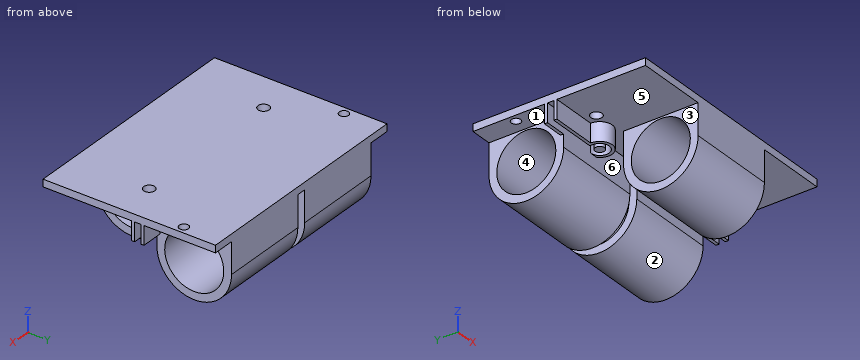
from build123d import *

# Parameters (mm, degrees)
SKETCH1_R              = 1.79994
SKETCH1_R_2            = 1.5
BOSS_EXTRUDE1_DEPTH    = 7
SKETCH2_W              = 75
SKETCH2_H              = 13.099999962
SKETCH2_R              = 2.6999438
SKETCH2_R_2            = 2.499995
SKETCH2_R_3            = 1.3498449
BOSS_EXTRUDE2_DEPTH    = 6.987999994
SKETCH2_3_R            = 2.6999438
SKETCH2_3_R_2          = 1.3498449
CUT_EXTRUDE1_DEPTH     = 2.5
SKETCH5_W              = 75
SKETCH5_H              = 13.099999962
CUT_EXTRUDE3_DEPTH     = 21.082
SKETCH6_W              = 75
SKETCH6_H              = 7
BOSS_EXTRUDE3_DEPTH    = 9.5
SKETCH8_W              = 75
SKETCH8_H              = 38.030205227
CUT_EXTRUDE4_DEPTH     = 4.666
SKETCH10_W             = 75
SKETCH10_H             = 2.334
BOSS_EXTRUDE5_DEPTH    = 25.000000038
SKETCH11_R             = 1.79994
CUT_EXTRUDE5_DEPTH     = 5
SKETCH15_W             = 44.653530321
SKETCH15_H             = 13.617301916
SKETCH15_W_2           = 11.728266088
SKETCH15_H_2           = 5.987537529
BOSS_EXTRUDE7_DEPTH    = 2.334
SKETCH16_R             = 9.5
BOSS_EXTRUDE9_DEPTH    = 29
SKETCH17_R             = 9.5
BOSS_EXTRUDE11_DEPTH   = 14.5
SKETCH18_W             = 6.99999997
SKETCH18_H             = 1
BOSS_EXTRUDE12_DEPTH   = 6
BOSS_EXTRUDE12_2_DEPTH = 6
SKETCH18_R             = 1.5
BOSS_EXTRUDE12_3_DEPTH = 6


with BuildPart() as part:
    # Sketch1 → Boss-Extrude1 (new body)
    with BuildSketch(Plane.XY):
        with BuildLine():
            Line((37.5, -10.5), (30, -10.5))
            ThreePointArc((30, -10.5), (25, -15.5), (20, -10.5))
            Line((20, -10.5), (5, -10.5))
            ThreePointArc((5, -10.5), (0, -15.5), (-5, -10.5))
            Line((-5, -10.5), (-20, -10.5))
            ThreePointArc((-20, -10.5), (-25, -15.5), (-30, -10.5))
            Line((-30, -10.5), (-37.5, -10.5))
            Line((-37.5, -10.5), (-37.5, 10.5))
            Line((-37.5, 10.5), (37.5, 10.5))
            Line((37.5, 10.5), (37.5, -10.5))
        make_face()
        with Locations((-25, -10.5)):
            Circle(SKETCH1_R, mode=Mode.SUBTRACT)
        with Locations((0, -10.5)):
            Circle(SKETCH1_R, mode=Mode.SUBTRACT)
        with Locations((25, -10.5)):
            Circle(SKETCH1_R, mode=Mode.SUBTRACT)
        with Locations((-35, 8)):
            Circle(SKETCH1_R_2, mode=Mode.SUBTRACT)
        with Locations(Location((-15, 8, 0), (0, 0, 180))):
            Circle(SKETCH1_R_2, mode=Mode.SUBTRACT)
        with Locations((-10, 8)):
            Circle(SKETCH1_R_2, mode=Mode.SUBTRACT)
        with Locations(Location((10, 8, 0), (0, 0, 180))):
            Circle(SKETCH1_R_2, mode=Mode.SUBTRACT)
        with Locations(Location((35, 8, 0), (0, 0, 180))):
            Circle(SKETCH1_R_2, mode=Mode.SUBTRACT)
        with Locations((15, 8)):
            Circle(SKETCH1_R_2, mode=Mode.SUBTRACT)
    extrude(amount=BOSS_EXTRUDE1_DEPTH)

    # Sketch2 → Boss-Extrude2 (add)
    # profile 1 of 7: a face of its own
    with BuildSketch(Plane(origin=(0, 2.24999999, 0), x_dir=(1, 0, 0), z_dir=(0, 1, 0))):
        with Locations((0, -13.549999981)):
            Rectangle(SKETCH2_W, SKETCH2_H)
        with Locations((31.0001404, -13.549999981)):
            Circle(SKETCH2_R, mode=Mode.SUBTRACT)
        with Locations((-31.0001404, -13.549999981)):
            Circle(SKETCH2_R, mode=Mode.SUBTRACT)
        with Locations(Location((-25, -13.549999981, 0), (0, 0, 180))):
            Circle(SKETCH2_R_2, mode=Mode.SUBTRACT)
        with Locations((-6.0001404, -13.549999981)):
            Circle(SKETCH2_R, mode=Mode.SUBTRACT)
        with Locations((6.0001404, -13.549999981)):
            Circle(SKETCH2_R, mode=Mode.SUBTRACT)
        with Locations(Location((0, -13.549999981, 0), (0, 0, 180))):
            Circle(SKETCH2_R_2, mode=Mode.SUBTRACT)
        with Locations((-18.9998596, -13.549999981)):
            Circle(SKETCH2_R, mode=Mode.SUBTRACT)
        with Locations(Location((25, -13.549999981, 0), (0, 0, 180))):
            Circle(SKETCH2_R_2, mode=Mode.SUBTRACT)
        with Locations((18.9998596, -13.549999981)):
            Circle(SKETCH2_R, mode=Mode.SUBTRACT)
    # profile 2 of 7: a face of its own
    with BuildSketch(Plane(origin=(0, 2.24999999, 0), x_dir=(1, 0, 0), z_dir=(0, 1, 0))):
        with Locations((-31.0001404, -13.549999981)):
            Circle(SKETCH2_R)
        with Locations(Location((-31.0001404, -13.549999981, 0), (0, 0, 180))):
            Circle(SKETCH2_R_3, mode=Mode.SUBTRACT)
    # profile 3 of 7: a face of its own
    with BuildSketch(Plane(origin=(0, 2.24999999, 0), x_dir=(1, 0, 0), z_dir=(0, 1, 0))):
        with Locations((-18.9998596, -13.549999981)):
            Circle(SKETCH2_R)
        with Locations(Location((-18.9998596, -13.549999981, 0), (0, 0, 180))):
            Circle(SKETCH2_R_3, mode=Mode.SUBTRACT)
    # profile 4 of 7: a face of its own
    with BuildSketch(Plane(origin=(0, 2.24999999, 0), x_dir=(1, 0, 0), z_dir=(0, 1, 0))):
        with Locations((-6.0001404, -13.549999981)):
            Circle(SKETCH2_R)
        with Locations(Location((-6.0001404, -13.549999981, 0), (0, 0, 180))):
            Circle(SKETCH2_R_3, mode=Mode.SUBTRACT)
    # profile 5 of 7: a face of its own
    with BuildSketch(Plane(origin=(0, 2.24999999, 0), x_dir=(1, 0, 0), z_dir=(0, 1, 0))):
        with Locations((6.0001404, -13.549999981)):
            Circle(SKETCH2_R)
        with Locations(Location((6.0001404, -13.549999981, 0), (0, 0, 180))):
            Circle(SKETCH2_R_3, mode=Mode.SUBTRACT)
    # profile 6 of 7: a face of its own
    with BuildSketch(Plane(origin=(0, 2.24999999, 0), x_dir=(1, 0, 0), z_dir=(0, 1, 0))):
        with Locations((18.9998596, -13.549999981)):
            Circle(SKETCH2_R)
        with Locations(Location((18.9998596, -13.549999981, 0), (0, 0, 180))):
            Circle(SKETCH2_R_3, mode=Mode.SUBTRACT)
    # profile 7 of 7: a face of its own
    with BuildSketch(Plane(origin=(0, 2.24999999, 0), x_dir=(1, 0, 0), z_dir=(0, 1, 0))):
        with Locations((31.0001404, -13.549999981)):
            Circle(SKETCH2_R)
        with Locations(Location((31.0001404, -13.549999981, 0), (0, 0, 180))):
            Circle(SKETCH2_R_3, mode=Mode.SUBTRACT)
    extrude(amount=-BOSS_EXTRUDE2_DEPTH)

    # Sketch2<3> → Cut-Extrude1 (cut)
    # profile 1 of 6: a face of its own
    with BuildSketch(Plane(origin=(0, 2.24999999, 0), x_dir=(1, 0, 0), z_dir=(0, 1, 0))):
        with Locations(Location((-31.0001404, -13.549999981, 0), (0, 0, 180))):
            Circle(SKETCH2_3_R)
        with Locations(Location((-31.0001404, -13.549999981, 0), (0, 0, 180))):
            Circle(SKETCH2_3_R_2, mode=Mode.SUBTRACT)
    # profile 2 of 6: a face of its own
    with BuildSketch(Plane(origin=(0, 2.24999999, 0), x_dir=(1, 0, 0), z_dir=(0, 1, 0))):
        with Locations(Location((-18.9998596, -13.549999981, 0), (0, 0, 180))):
            Circle(SKETCH2_3_R)
        with Locations(Location((-18.9998596, -13.549999981, 0), (0, 0, 180))):
            Circle(SKETCH2_3_R_2, mode=Mode.SUBTRACT)
    # profile 3 of 6: a face of its own
    with BuildSketch(Plane(origin=(0, 2.24999999, 0), x_dir=(1, 0, 0), z_dir=(0, 1, 0))):
        with Locations(Location((-6.0001404, -13.549999981, 0), (0, 0, 180))):
            Circle(SKETCH2_3_R)
        with Locations(Location((-6.0001404, -13.549999981, 0), (0, 0, 180))):
            Circle(SKETCH2_3_R_2, mode=Mode.SUBTRACT)
    # profile 4 of 6: a face of its own
    with BuildSketch(Plane(origin=(0, 2.24999999, 0), x_dir=(1, 0, 0), z_dir=(0, 1, 0))):
        with Locations(Location((6.0001404, -13.549999981, 0), (0, 0, 180))):
            Circle(SKETCH2_3_R)
        with Locations(Location((6.0001404, -13.549999981, 0), (0, 0, 180))):
            Circle(SKETCH2_3_R_2, mode=Mode.SUBTRACT)
    # profile 5 of 6: a face of its own
    with BuildSketch(Plane(origin=(0, 2.24999999, 0), x_dir=(1, 0, 0), z_dir=(0, 1, 0))):
        with Locations(Location((18.9998596, -13.549999981, 0), (0, 0, 180))):
            Circle(SKETCH2_3_R)
        with Locations(Location((18.9998596, -13.549999981, 0), (0, 0, 180))):
            Circle(SKETCH2_3_R_2, mode=Mode.SUBTRACT)
    # profile 6 of 6: a face of its own
    with BuildSketch(Plane(origin=(0, 2.24999999, 0), x_dir=(1, 0, 0), z_dir=(0, 1, 0))):
        with Locations(Location((31.0001404, -13.549999981, 0), (0, 0, 180))):
            Circle(SKETCH2_3_R)
        with Locations(Location((31.0001404, -13.549999981, 0), (0, 0, 180))):
            Circle(SKETCH2_3_R_2, mode=Mode.SUBTRACT)
    extrude(amount=-CUT_EXTRUDE1_DEPTH, mode=Mode.SUBTRACT)

    # Sketch5 → Cut-Extrude3 (cut)
    with BuildSketch(Plane(origin=(0, 2.24999999, 0), x_dir=(1, 0, 0), z_dir=(0, 1, 0))):
        with Locations((0, -13.549999981)):
            Rectangle(SKETCH5_W, SKETCH5_H)
    extrude(amount=-CUT_EXTRUDE3_DEPTH, mode=Mode.SUBTRACT)

    # Sketch6 → Boss-Extrude3 (add)
    with BuildSketch(Plane(origin=(0, 10.5, 0), x_dir=(1, 0, 0), z_dir=(0, 1, 0))):
        with Locations((0, -3.5)):
            Rectangle(SKETCH6_W, SKETCH6_H)
    extrude(amount=BOSS_EXTRUDE3_DEPTH)

    # Sketch8 → Cut-Extrude4 (cut)
    with BuildSketch(Plane(origin=(0, 0, 0), x_dir=(-1, 0, 0), z_dir=(0, 0, -1))):
        with Locations((0, 0.984897387)):
            Rectangle(SKETCH8_W, SKETCH8_H)
    extrude(amount=-CUT_EXTRUDE4_DEPTH, mode=Mode.SUBTRACT)

    # Sketch10 → Boss-Extrude5 (add)
    with BuildSketch(Plane(origin=(0, -35.500000038, 0), x_dir=(-1, 0, 0), z_dir=(0, -1, 0))):
        with Locations((0, -5.833)):
            Rectangle(SKETCH10_W, SKETCH10_H)
    extrude(amount=-BOSS_EXTRUDE5_DEPTH)

    # Sketch11 → Cut-Extrude5 (cut)
    with BuildSketch(Plane(origin=(0, 0, 4.666), x_dir=(-1, 0, 0), z_dir=(0, 0, -1))):
        with Locations((-25, -10.5)):
            Circle(SKETCH11_R)
        with Locations((0, -10.5)):
            Circle(SKETCH11_R)
        with Locations((25, -10.5)):
            Circle(SKETCH11_R)
    extrude(amount=-CUT_EXTRUDE5_DEPTH, mode=Mode.SUBTRACT)

    # Sketch15 → Boss-Extrude7 (add)
    with BuildSketch(Plane.XY.offset(7)):
        with Locations((1.804442165, 8.803924913)):
            Rectangle(SKETCH15_W, SKETCH15_H)
        with Locations((-1.501191344, -11.287680254)):
            Rectangle(SKETCH15_W_2, SKETCH15_H_2)
    extrude(amount=-BOSS_EXTRUDE7_DEPTH)


with BuildPart() as body_2:
    # Sketch16 → Boss-Extrude9 (new body)
    with BuildSketch(Plane(origin=(30.50000003, 0, 0), x_dir=(0, 0, -1), z_dir=(1, 0, 0))):
        with BuildLine():
            Line((-4.666, 9.5), (-4.666, 6.5))
            Line((-4.666, 6.5), (-4.666, -4))
            Line((-4.666, -4), (5.334, -4))
            ThreePointArc((5.334, -4), (17.334, 8), (5.334, 20))
            Line((5.334, 20), (-4.666, 20))
            Line((-4.666, 20), (-4.666, 9.5))
        make_face()
        with Locations((5.334, 8)):
            Circle(SKETCH16_R, mode=Mode.SUBTRACT)
    extrude(amount=-BOSS_EXTRUDE9_DEPTH)


with BuildPart() as body_3:
    # Mirror1: mirrored copy
    add(body_2.part.mirror(Plane(origin=(0, 0, 0), x_dir=(0, 0, 1), z_dir=(1, 0, 0))))

    # Combine1: union body 2, part
    add(body_2.part)
    add(part.part)

    # Sketch17 → Boss-Extrude11 (add, symmetric)
    with BuildSketch(Plane(origin=(0, 0, 0), x_dir=(0, 0, -1), z_dir=(1, 0, 0))):
        with BuildLine():
            Line((5.334, -35.500000038), (-4.666, -35.500000038))
            Line((-4.666, -35.500000038), (-4.666, -11.500000038))
            Line((-4.666, -11.500000038), (5.334, -11.500000038))
            ThreePointArc((5.334, -11.500000038), (17.334, -23.500000038), (5.334, -35.500000038))
        make_face()
        with Locations(Location((5.334, -23.500000038, 0), (0, 0, 180))):
            Circle(SKETCH17_R, mode=Mode.SUBTRACT)
    extrude(amount=BOSS_EXTRUDE11_DEPTH, both=True)


with BuildPart() as body_2_2:
    # Sketch18 → Boss-Extrude12 (new body)
    with BuildSketch(Plane(origin=(0, 0, 4.666), x_dir=(-1, 0, 0), z_dir=(0, 0, -1))):
        with Locations((-34.000000015, -3.5)):
            Rectangle(SKETCH18_W, SKETCH18_H)
    extrude(amount=BOSS_EXTRUDE12_DEPTH)


with BuildPart() as body_3_2:
    # Sketch18 → Boss-Extrude12 2 (new body)
    with BuildSketch(Plane(origin=(0, 0, 4.666), x_dir=(-1, 0, 0), z_dir=(0, 0, -1))):
        with BuildLine():
            Line((-16.114044259, -4), (-18.762606579, -4))
            ThreePointArc((-18.762606579, -4), (-16.636024525, -9.134023236), (-21.770047761, -7.007441182))
            Line((-21.770047761, -7.007441182), (-21.770047761, -6))
            Line((-21.770047761, -6), (-37.5, -6))
            Line((-37.5, -6), (-37.5, -7))
            Line((-37.5, -7), (-22.770047761, -7))
            Line((-22.770047761, -7), (-22.770047761, -7.007441182))
            ThreePointArc((-22.770047761, -7.007441182), (-17.112511564, -10.659395628), (-16.114044259, -4))
        make_face()
    extrude(amount=BOSS_EXTRUDE12_2_DEPTH)


with BuildPart() as body_4:
    # Sketch18 → Boss-Extrude12 3 (new body)
    with BuildSketch(Plane(origin=(0, 0, 4.666), x_dir=(-1, 0, 0), z_dir=(0, 0, -1))):
        with Locations((-18.762606579, -7.007441182)):
            Circle(SKETCH18_R)
    extrude(amount=BOSS_EXTRUDE12_3_DEPTH)


with BuildPart() as body_5:
    # Mirror2: mirrored copy
    add(body_3_2.part.mirror(Plane(origin=(0, 0, 0), x_dir=(0, 0, 1), z_dir=(1, 0, 0))))


with BuildPart() as body_6:
    # Mirror2 2: mirrored copy
    add(body_4.part.mirror(Plane(origin=(0, 0, 0), x_dir=(0, 0, 1), z_dir=(1, 0, 0))))


with BuildPart() as body_7:
    # Mirror2 3: mirrored copy
    add(body_2_2.part.mirror(Plane(origin=(0, 0, 0), x_dir=(0, 0, 1), z_dir=(1, 0, 0))))


with BuildPart() as body_5_1:
    add(body_5.part)

    # Combine2: union body 7, body 2 2, body 4, body 3 2, body 3, body 6
    add(body_7.part)
    add(body_2_2.part)
    add(body_4.part)
    add(body_3_2.part)
    add(body_3.part)
    add(body_6.part)


solid = body_5_1.part
Source: CAD feature listing. Evaluate the final solid. Frame: model axes, mm. Face numbers are marked on the shaded views. A direction names the side the tool comes from. Round coordinates to 2 decimals unless told otherwise and drop trailing zeros. Loops run counter-clockwise (first coordinate to the right, second up) from the corner with the lowest first, then second, coordinate; pieces in that order, holes last.
Q1. Ray query, line 1 (X direction, y = 8, z = 5.65); line 2 (Y direction, x = 25, z = 5); line 3 (X direction, y = 18.5, z = 4). Return the intervals inside material, ascending.
Q2. Section B-B, the plane y = 8. Return loops of the section in (x, z).
Q3. Access query for the marked faces 1 and 2. Directions: +Z, -Z, +X, -X, +Y, -Y. A direction counts if a zero-diameter tool reaches every point of the face in a straight line with its end or side. Return the directions, or none.
Q4. Section D-D, the plane z = -9.5. Return loops of the section in (x, y).
Q5. Mould query, pull axis X, two halves, no side actions, for the marked faces 3, 4, 5 and 6. Classes: pulls with the +X half, pulls with the -X half, needs draft (parallel to the pull), parting line crosses it, or undercut.
Q6. First-contact query: P1, Ø5, axis at x = 31.5, z = 2, coming from the -Y side; P2, Ø1, axis at y = -16, z = 1.5, coming from the +X side; P3, Ø2.5, axis at x = -18.5, y = -7, coming from the -Z side. Flat tips, straight axial feed; report the tip coordinate or a pass-through.
Q7. Section A-A, the plane x = -25. Return loops of the section in (y, z), plus the area to 3 significant figures.
Q8. Section C-C, the plane x = -35. Return loops of the section in (y, z), plus the area to 3 significant figures.
Solutions:
1. line 1: x = -37.5 to -36.5, -33.5 to 33.5, 36.5 to 37.5
1. line 2: y = -35.5 to -12.3, -8.7 to 20
1. line 3: x = -30.5 to -1.5, 1.5 to 30.5
2. outline: (-37.5, 4.67) - (-36.5, 4.67) - (-36.5, 7) - (-37.5, 7) - close; (-33.5, 4.67) - (-30.5, 4.67) - (-30.5, 4.17) - (-1.5, 4.17) - (-1.5, 4.67) - (1.5, 4.67) - (1.5, 4.17) - (30.5, 4.17) - (30.5, 4.67) - (33.5, 4.67) - (33.5, 7) - (-33.5, 7) - close; (-30.5, -17.33) - (-1.5, -17.33) - (-1.5, -14.83) - (-30.5, -14.83) - close; (1.5, -17.33) - (30.5, -17.33) - (30.5, -14.83) - (1.5, -14.83) - close; (36.5, 4.67) - (37.5, 4.67) - (37.5, 7) - (36.5, 7) - close
3. face 1: -Z, -X, +Y
3. face 2: -Z, +X, -X
4. outline: (-30.5, -3.25) - (-1.5, -3.25) - (-1.5, -0.54) - (-30.5, -0.54) - close; (-30.5, 16.54) - (-1.5, 16.54) - (-1.5, 19.25) - (-30.5, 19.25) - close; (-14.5, -34.75) - (14.5, -34.75) - (14.5, -32.04) - (-14.5, -32.04) - close; (-14.5, -14.96) - (14.5, -14.96) - (14.5, -12.25) - (-14.5, -12.25) - close; (1.5, -3.25) - (30.5, -3.25) - (30.5, -0.54) - (1.5, -0.54) - close; (1.5, 16.54) - (30.5, 16.54) - (30.5, 19.25) - (1.5, 19.25) - close
5. face 3: pulls with the -X half
5. face 4: needs draft
5. face 5: undercut
5. face 6: undercut
6. P1: stops at y = -7
6. P2: stops at x = 14.5
6. P3: stops at z = -1.33
7. outline: (-35.5, 4.67) - (-12.3, 4.67) - (-12.3, 7) - (-35.5, 7) - close; (-8.7, 4.67) - (-7, 4.67) - (-7, -1.33) - (-6, -1.33) - (-6, 4.67) - (-4, 4.67) - (-4, -5.33) arc R12 ccw to (20, -5.33) - (20, 7) - (-8.7, 7) - close; hole circle Ø19 at (8, -5.33)
7. area: 310 mm2
8. outline: (-35.5, 4.67) - (-7, 4.67) - (-7, -1.33) - (-6, -1.33) - (-6, 4.67) - (-4, 4.67) - (-4, -1.33) - (-3, -1.33) - (-3, 4.67) - (6.5, 4.67) - (6.5, 7) - (-35.5, 7) - close; (9.5, 4.67) - (20, 4.67) - (20, 7) - (9.5, 7) - close
8. area: 135 mm2
